Verification items for the finished model (mm, model axes). Give positions to 0.01 mm unless a question says otherwise; leave off trailing zeros. Order: outer loops, then holes, each group sorted by start corner. A loop starts at its lowest first (then second) coordinate and runs counter-clockwise, first axis right, second up. Notation, with made-up numbers: (-33, 88) -> (-17, 88) arc R23 ccw to (-17, 124) -> close; hole circle Ø5 at (7, -7.75). An arc over 180 degrees is marked (long way). One line per question, with ' | ' between items. Start each with the question number.
Q1. Material ranges on probe 1 along X at (y, z) = (30, -34.5); probe 2 along Y at (x, z) = (211.5, -33); probe 3 along Z at (x, y) = (193, 8.5), recorded low to high. Write a range as [from, to].
Q2. Section check B-B on x = 71.5. Record the cut outline in (y, z), plus the area to 3 significant figures.
Q3. Section check A-A on z = 10. Record the cut outline in (x, y), plus the area to 3 significant figures.
Q4. Go/stop test with flat-tipped pins: pin 1 (8 mm diameter, centred on x = 501.5, z = -7.5, fed in from +Y); pin 2 (4 mm diameter, centred on x = 214.5, y = 11.5, fed in from +Z); pin 3 (1 mm diameter, centred on x = 461, z = 26, fed in from +Y). Record where each tip stops, or that it passes through.
Q5. Section check C-C on z = -27.5. Record the cut outline in (x, y).
from build123d import *

# Parameters (mm, degrees)
BOSS_EXTRUDE1_START = 100
SKETCH4_R           = 50
BOSS_EXTRUDE1_DEPTH = 100


with BuildPart() as part:
    # Sketch3 → Revolve1 (revolve)
    with BuildSketch(Plane.XY, mode=Mode.PRIVATE) as revolve1_sk:
        Polygon((0, 0), (0, 50), (2.676183962, 50), (636.2, 50), (636.2, 37.5), (661.2, 37.5), (661.2, 50), (700, 50), (700, 0), align=None)
    revolve(revolve1_sk.sketch.rotate(Axis((0, 0, 0), (1, 0, 0)), 90), axis=Axis((0, 0, 0), (1, 0, 0)))

    # Sketch4 → Boss-Extrude1 (add)
    with BuildSketch(Plane(origin=(700, 0, 0), x_dir=(0, 0, -1), z_dir=(1, 0, 0)).offset(BOSS_EXTRUDE1_START)):
        with Locations(Location((0, 0, 0), (0, 0, 180))):
            Circle(SKETCH4_R)
    extrude(amount=-BOSS_EXTRUDE1_DEPTH)


solid = part.part
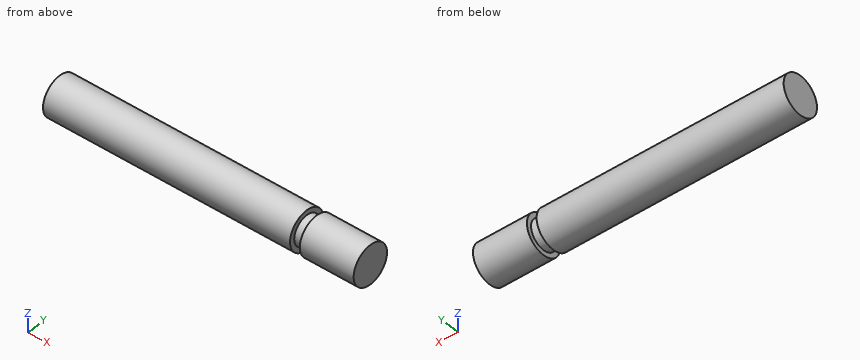
Filled in:
1) probe 1: [0, 636.2], [661.2, 800] | probe 2: [-37.56, 37.56] | probe 3: [-49.27, 49.27]
2) outline: circle Ø100 at (0, 0) | area: 7,850 mm²
3) outline: (0, -48.99) -> (636.2, -48.99) -> (636.2, -36.14) -> (661.2, -36.14) -> (661.2, -48.99) -> (800, -48.99) -> (800, 48.99) -> (661.2, 48.99) -> (661.2, 36.14) -> (636.2, 36.14) -> (636.2, 48.99) -> (0, 48.99) -> close | area: 77,700 mm²
4) pin 1: y = 49.88 | pin 2: z = 49.09 | pin 3: y = 43.01
5) outline: (0, -41.76) -> (636.2, -41.76) -> (636.2, -25.5) -> (661.2, -25.5) -> (661.2, -41.76) -> (800, -41.76) -> (800, 41.76) -> (661.2, 41.76) -> (661.2, 25.5) -> (636.2, 25.5) -> (636.2, 41.76) -> (0, 41.76) -> close
